Here's the drawing with two shaded views (mm, measured from the low corner). I have some questions. A direction names the side the tool comes from. Round coordinates to 2 decimals unless told otherwise and drop trailing zeros. Order: outer loops, then holes, each group sorted by start corner. A loop starts at its lowest first (then second) coordinate and runs counter-clockwise, first axis right, second up. Notation, with made-up numbers: (-15, 6.25) -> (-10, 6.25) arc R22 ccw to (-10, 14.25) -> close; hole circle Ø8 at (54, -16.75). An arc over 180 degrees is marked (long way). One line per question, with ' | ' between items.
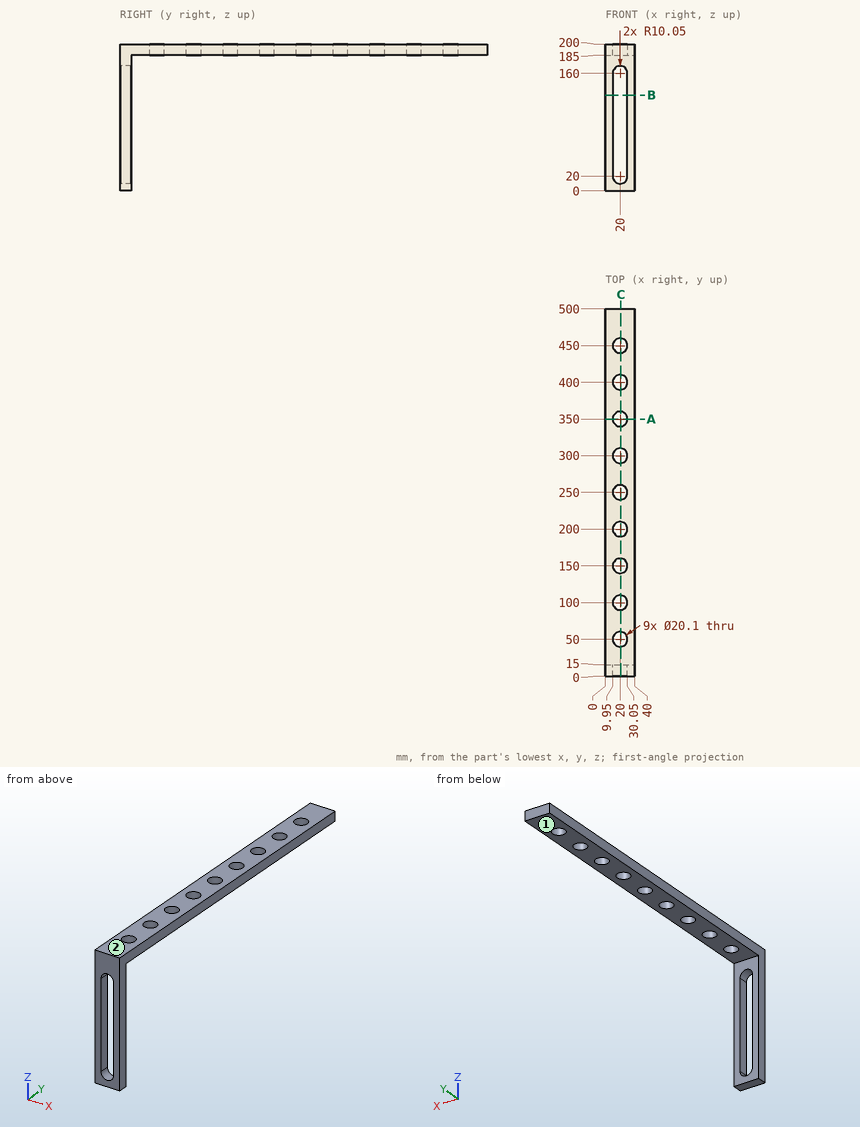
1. I need wall thicknesses on probe 1 along Z at (x, y) = (13, 286); probe 2 along Y at (x, z) = (38, 117). Which ranges of each line are inside material? Lowest first, please.
From the geometry:
probe 1: z = 185 to 200 | probe 2: y = 0 to 15
2. I'm going to push flat-ended pins straight in: pin 1 (12 mm diameter, centred on x = 25, z = 101, fed in from +Y); pin 2 (23 mm diameter, centred on x = 20, y = 250, fed in from -Z); pin 3 (12 mm diameter, centred on x = 31, z = 68.5, fed in from -Y). Where does each tip first touch, or does it pass through?
From the geometry:
pin 1: stops at y = 15 | pin 2: stops at z = 185 | pin 3: stops at y = 0
3. I want a section at A-A on y = 350. List the corners of the cut face in (x, z) for me.
From the geometry:
outline: (0, 185) -> (9.95, 185) -> (9.95, 200) -> (0, 200) -> close; (30.05, 185) -> (40, 185) -> (40, 200) -> (30.05, 200) -> close
4. I want a section at C-C on x = 21. Count the separate pieces of the cut face and the enclosed holes in it, and give its area (3 significant figures).
From the geometry:
separate pieces: 11 | enclosed holes: 0 | area: 5,170 mm²
5. I want a section at B-B on z = 130.5. List the corners of the cut face in (x, y) for me, and give its area (4 significant figures).
From the geometry:
outline: (0, 0) -> (9.95, 0) -> (9.95, 15) -> (0, 15) -> close; (30.05, 0) -> (40, 0) -> (40, 15) -> (30.05, 15) -> close | area: 298.5 mm²
6. On a 3-axis mill with a long thin cutter (end or side, diameter ignored), from which of +Z, -Z, +X, -X, +Y, -Y can I reach the whole of each face in a straight line? I mean the marked faces 1 and 2. Say none if no direction works.
From the geometry:
face 1: -Z, +X, -X, +Y | face 2: +Z, +X, -X, +Y, -Y
